CAD build for the part. Positions are in the model's coordinates, mm. Face numbers are marked on the shaded views. A direction names the side the tool comes from. Give positions to 0.01 mm unless a question says otherwise; leave off trailing zeros. Loops run counter-clockwise (first coordinate to the right, second up) from the corner with the lowest first, then second, coordinate; pieces in that order, holes last. Notation, with made-up numbers: (33, -38.75) - (89, -38.75) arc R15 ccw to (89, -23.75) - close; hole circle Ø3 at (18, 35.5). An arc over 180 degrees is marked (long way). Return JSON: item names as keys, results as strings.
from build123d import *

# Parameters (mm, degrees)
SKETCH_1_W      = 88.3
SKETCH_1_H      = 57.77
EXTRUDE_1_DEPTH = 18.9
SKETCH_2_W      = 13.76
SKETCH_2_H      = 17
EXTRUDE_2_DEPTH = 48
SKETCH_3_W      = 10.848746397
SKETCH_3_H      = 3.037648992
EXTRUDE_3_DEPTH = 45


with BuildPart() as part:
    # Эскиз1 → Бобышка-Вытянуть1 (new body)
    with BuildSketch(Plane(origin=(0, 0, 0), x_dir=(1, 0, 0), z_dir=(0, 1, 0))):
        with Locations((-24.816331195, -7.343762185)):
            Rectangle(SKETCH_1_W, SKETCH_1_H)
    extrude(amount=EXTRUDE_1_DEPTH)

    # Эскиз2 → Бобышка-Вытянуть2 (add)
    with BuildSketch(Plane.ZY.offset(68.966331195)):
        with Locations((-13.462732009, 9.722786208)):
            Rectangle(SKETCH_2_W, SKETCH_2_H)
    extrude(amount=EXTRUDE_2_DEPTH)

    # Эскиз3 → Бобышка-Вытянуть3 (add)
    with BuildSketch(Plane(origin=(0, 0, -21.541237815), x_dir=(-1, 0, 0), z_dir=(0, 0, -1))):
        with Locations((-6.878820548, 3.164454924)):
            Rectangle(SKETCH_3_W, SKETCH_3_H)
    extrude(amount=EXTRUDE_3_DEPTH)


solid = part.part
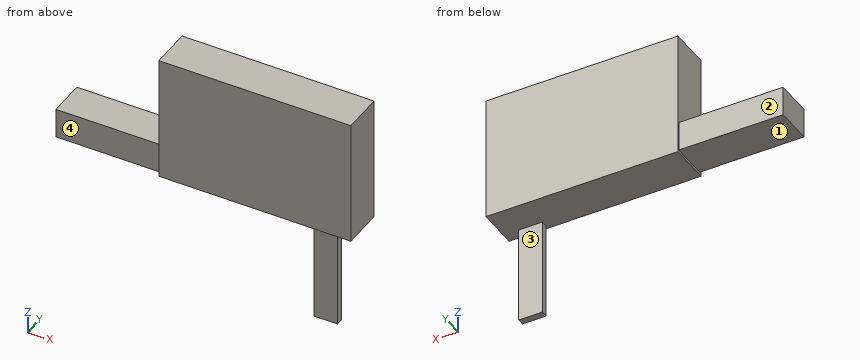
1. Drop flat-ended pins along their axis: P1, Ø4, axis at x = -97, y = 11.5, coming from the +Z side; P2, Ø1.5, axis at x = -60, y = 7, coming from the -Z side; P3, Ø8.5, axis at x = 5.5, z = -35.5, coming from the -Y side. Give the stop position or say it passes through.
Values follow:
{"P1": "stops at z = -6.58", "P2": "stops at z = -21.54", "P3": "stops at y = 1.65"}
2. Which spindle directions (+Z, -Z, +X, -X, +Y, -Y) get a long thin tool onto all of the face, cutting with end or side? Do the marked faces 1, 2, 3 and 4. Say none if no direction does.
Values follow:
{"face 1": "-Z, -X, +Y, -Y", "face 2": "+Z, -Z, -X, +Y", "face 3": "-Z, +X, -X, +Y", "face 4": "+Z, -Z, -X, -Y"}
3. Cut at A-A, the plane y = 13.5. Write the cut outline in (x, z), plus the area to 3 significant figures.
Values follow:
{"outline": "(-116.97, -20.34) - (-68.97, -20.34) - (-68.97, -21.54) - (19.33, -21.54) - (19.33, 36.23) - (-68.97, 36.23) - (-68.97, -6.58) - (-116.97, -6.58) - close", "area": "5,760 mm²"}
4. Cut at B-B, the plane x = -20. Write the cut outline in (y, z), plus the area to 3 significant figures.
Values follow:
{"outline": "(0, -21.54) - (18.9, -21.54) - (18.9, 36.23) - (0, 36.23) - close", "area": "1,090 mm²"}
5. Drill centre lines: probe 1 along Z at (x, y) = (-94, 14.25); probe 2 along X at (y, z) = (5, 17); probe 3 along Z at (x, y) = (-1, 17.25). Where is each one in solid material? Low to high.
Values follow:
{"probe 1": "z = -20.34 to -6.58", "probe 2": "x = -68.97 to 19.33", "probe 3": "z = -21.54 to 36.23"}
6. Cut at C-C, the plane z = -2. Write the cut outline in (x, y).
Values follow:
{"outline": "(-68.97, 0) - (19.33, 0) - (19.33, 18.9) - (-68.97, 18.9) - close"}
